The model under review builds one solid part; all positions refer to its coordinate system, in mm. Coordinates: 2 decimals unless noted, no trailing zeros.
```python
from build123d import *

# Parameters (mm, degrees)
F0_W     = 103.4416258335
F0_H     = 190.3689950705
F1_DEPTH = 20
F3_D     = 5.5
F4_SIZE  = 3
F6_D     = 8.8


# Not quite as in the source:
# - a feature names something its author has since deleted; it is built from what else it names


with BuildPart() as f1:
    # F0 (on Top) → F1 (new body)
    with BuildSketch(Plane.XY):
        with Locations((-51.7208129168, 95.1844975352)):
            Rectangle(F0_W, F0_H)
    extrude(amount=F1_DEPTH)

    # F3 (through all)
    with Locations(Plane.XY.offset(20)):
        with Locations((-20, 20), (-83.82, 167.386), (-20.066, 167.64), (-80.264, 22.352)):
            Hole(F3_D / 2)

    # F4
    f4_edges = [f1.edges().sort_by_distance(p)[0] for p in [
        (-51.720813, 0, 20),
        (-103.441626, 95.184498, 20),
        (0, 95.184498, 20),
        (-51.720813, 190.368995, 20),
        (-83.014, 22.352, 20),
        (-22.75, 20, 20),
        (-86.57, 167.386, 20),
        (-22.816, 167.64, 20),
    ]]
    chamfer(f4_edges, length=F4_SIZE)

    # F6 (through all)
    with Locations(Plane.XY.offset(20)):
        with Locations((-49.0952916443, 93.7389880419)):
            Hole(F6_D / 2)


solid = f1.part
```
Item 1: Take a section at A-A, the plane x = -20. Count the separate pieces of the cut face and the enclosed holes in it, plus the area to 3 significant figures.
Solved:
separate pieces: 3
enclosed holes: 0
area: 3,560 mm2
Item 2: Mouldability with a two-part tool opening along X and no side actions: class faces 1 (the face through (-52, 0, 8)), 2 (the face through (-17.866, 21.957, 17.146)), 3 (the face through (0, 94, 8)) as pulls with the +X half, pulls with the -X half, needs draft (parallel to the pull), parting line crosses it, or undercut.
Solved:
face 1: needs draft
face 2: undercut
face 3: pulls with the +X half
Item 3: To check wall thickness, follow line 1 along X through (y, z) = (167.64, 7); line 2 along Y through (x, z) = (-20, 9.5); line 3 along Y through (x, z) = (-22, 7.75). State the ranges of each line that lie inside material, in increasing order.
Solved:
line 1: x = -103.44 to -86.56, -81.08 to -22.82, -17.32 to 0
line 2: y = 0 to 17.25, 22.75 to 164.89, 170.39 to 190.37
line 3: y = 0 to 18.11, 21.89 to 165.68, 169.6 to 190.37
Item 4: For pin 1 (6.5 mm diameter, centred on x = -80.264, y = 22.352, fed in from +Z), flat-tipped, find the tip position at first contact; note if it passes through.
Solved:
pin 1: stops at z = 17.5
